Geometry: see drawing. Coordinates: mm, zero at the bounding-box minimum. A direction names the side the tool comes from. Coordinates: 2 decimals unless noted, no trailing zeros. Loops run counter-clockwise (first coordinate to the right, second up) from the corner with the lowest first, then second, coordinate; pieces in that order, holes last. Notation, with made-up numbers: (-21, 85) -> (3, 85) arc R23 cw to (3, 108) -> close; hole circle Ø2 at (60.5, 52.5). An arc over 180 degrees is marked (long way). Put each result on its own line as item: value. Start each with the question number.
1) Pull-direction query (Y, two-part tool) for the marked faces 1, 2 and 3; classes: pulls with the +Y half, pulls with the -Y half, needs draft (parallel to the pull), parting line crosses it, or undercut.
2) Cut plane C-C (y = 28.5). Return the cut outline in (x, z) (1 decimal), plus the area to 3 significant figures.
3) Contact query for flat-ended pins moving along their axis: P1, Ø3.5, axis at x = 5.5, y = 31, coming from the -Z side; P2, Ø1.5, axis at x = 7, z = 27.5, coming from the +Y side; P3, Ø5, axis at x = 5.5, z = 52.5, coming from the -Y side. Output: stop coordinate, or through.
4) Cut plane B-B (x = 5.75). Return the cut outline in (y, z) (1 decimal).
5) Material intervals for L1, parallel to Z at x = 1.75, y = 25 (1 decimal); L2, parallel to Y at x = 1, z = 35 (1 decimal); L3, parallel to Z at x = 2, y = 38 (1 decimal), sorted ascending.
6) Cut plane D-D (z = 24.5). Return the cut outline in (x, y) (1 decimal).
7) Cut plane A-A (x = 1.25). Return the cut outline in (y, z) (1 decimal), plus the area to 3 significant figures.
8) Set-up query: the marked faces 4, 5, 6 and 7. Return all of +Z, -Z, +X, -X, +Y, -Y with unobstructed straight access to the full face (end or side cutting, diameter ignored); none if empty.
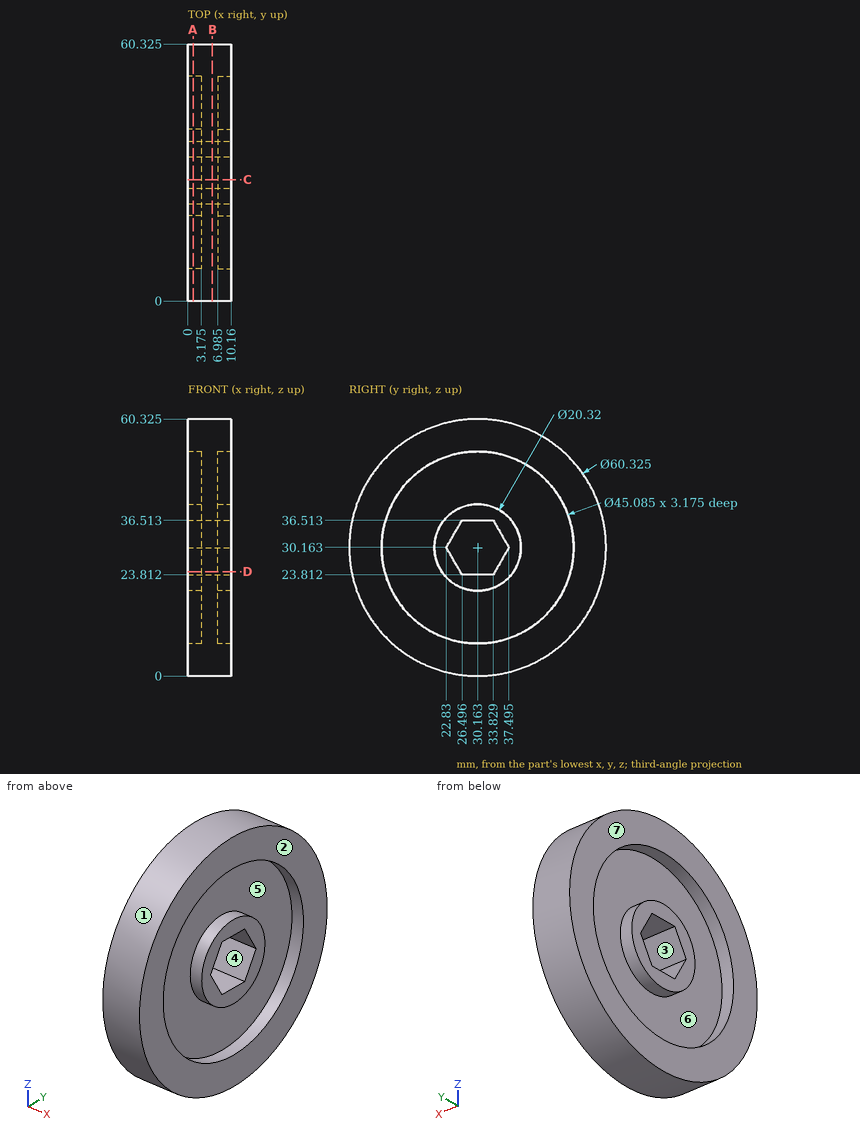
Results found:
1. face 1: parting line crosses it
1. face 2: needs draft
1. face 3: undercut
2. outline: (0, 0) -> (10.2, 0) -> (10.2, 7.7) -> (7, 7.7) -> (7, 20.1) -> (10.2, 20.1) -> (10.2, 23.8) -> (0, 23.8) -> (0, 20.1) -> (3.2, 20.1) -> (3.2, 7.7) -> (0, 7.7) -> close; (0, 36.5) -> (10.2, 36.5) -> (10.2, 40.2) -> (7, 40.2) -> (7, 52.6) -> (10.2, 52.6) -> (10.2, 60.3) -> (0, 60.3) -> (0, 52.6) -> (3.2, 52.6) -> (3.2, 40.2) -> (0, 40.2) -> close
2. area: 325 mm2
3. P1: stops at z = 0
3. P2: stops at y = 60.26
3. P3: stops at y = 7.44
4. outline: circle Ø60.3 at (30.2, 30.2); hole (22.8, 30.2) -> (26.5, 23.8) -> (33.8, 23.8) -> (37.5, 30.2) -> (33.8, 36.5) -> (26.5, 36.5) -> close
5. L1: z = 0.4 to 8.2, 21.4 to 26.4, 33.9 to 38.9, 52.1 to 59.9
5. L2: y = 0.4 to 8.1, 21.2 to 25.6, 34.7 to 39.1, 52.2 to 59.9
5. L3: z = 1 to 9, 23.7 to 36.6, 51.3 to 59.3
6. outline: (0, 0.5) -> (10.2, 0.5) -> (10.2, 8.3) -> (7, 8.3) -> (7, 21.7) -> (10.2, 21.7) -> (10.2, 26.1) -> (0, 26.1) -> (0, 21.7) -> (3.2, 21.7) -> (3.2, 8.3) -> (0, 8.3) -> close; (0, 34.2) -> (10.2, 34.2) -> (10.2, 38.6) -> (7, 38.6) -> (7, 52) -> (10.2, 52) -> (10.2, 59.8) -> (0, 59.8) -> (0, 52) -> (3.2, 52) -> (3.2, 38.6) -> (0, 38.6) -> close
7. outline: circle Ø60.3 at (30.2, 30.2); circle Ø20.3 at (30.2, 30.2); hole circle Ø45.1 at (30.2, 30.2); hole (22.8, 30.2) -> (26.5, 23.8) -> (33.8, 23.8) -> (37.5, 30.2) -> (33.8, 36.5) -> (26.5, 36.5) -> close
7. area: 1,450 mm2
8. face 4: +X, -X
8. face 5: +X
8. face 6: -X
8. face 7: +Z, -Z, -X, +Y, -Y
